Geometry: final body of the model. Coordinates: model frame, mm. A direction names the side the tool comes from. Round coordinates to 2 decimals unless told otherwise and drop trailing zeros. Order: outer loops, then holes, each group sorted by start corner. A loop starts at its lowest first (then second) coordinate and runs counter-clockwise, first axis right, second up. Notation, with made-up numbers: (-12, 30.25) - (33, 30.25) arc R21 ccw to (33, 52.25) - close; hole circle Ø5 at (9, -9.5). An arc over 180 degrees is marked (long way). Put each result on its own line as item: value. Start each with the question number.
(1) Pin query (flat end, axial travel): P1, Ø1.5, axis at x = 21, y = -4, coming from the -Z side; P2, Ø10.5, axis at x = 65.2, z = 33, coming from the -Y side; P3, Ø4, axis at x = 17, z = 40.5, coming from the -Y side; P4, Ø5, axis at x = 39.8, z = 33, coming from the -Y side (3 decimals). Return the tip coordinate at first contact, or that it passes through.
(2) Section C-C (z = 17.5). Output: boundary loops of the cut face in (x, y).
(3) Material intervals for L1, parallel to Y at x = 27.5, z = -1; L2, parallel to Z at x = 65, y = 5; L3, parallel to X at y = 5, z = 34, sorted ascending. Write a range as [from, to].
(4) Access query for faces 4 (the face through (1, 8.05, 1)), 5 (the face through (40, 14, 27.4)), 6 (the face through (1, 13, -13)). Directions: +Z, -Z, +X, -X, +Y, -Y. A direction counts if a zero-diameter tool reaches every point of the face in a straight line with its end or side. Return the directions, or none.
(5) Pull-direction query (X, two-part tool) for faces 1 (the face through (1, 1, 13)), 2 (the face through (70.072, 14.499, 30.239)), 3 (the face through (-90, 3, 24)); classes: released by +X, released by -X, zero draft, split by the parting line, or undercut.
(6) Section A-A (z = -5). Output: boundary loops of the cut face in (x, y).
from build123d import *

# Parameters (mm, degrees)
F1_DEPTH = 90
F2_W     = 6
F2_H     = 61
F3_DEPTH = 5
F4_R     = 3.25
F5_DEPTH = 30.001
F7_DEPTH = 7
F8_SIZE  = 0.99999
F9_SIZE  = 1


# Not quite as in the source:
# - a fillet or chamfer is up to 0.001 mm smaller than in the source, because OpenCascade refuses the exact size


with BuildPart() as f1:
    # F0 (on Right) → F1 (new body, symmetric)
    with BuildSketch(Plane.YZ):
        Polygon((-6.05, 13), (8.05, 13), (8.05, -13), (17.95, -13), (17.95, 48), (-12.05, 48), (-12.05, -13), (-8.05, -13), (-8.05, 14), (-6.05, 14), align=None)
    extrude(amount=F1_DEPTH, both=True)

    # F2 (on face) → F3 (join)
    with BuildSketch(Plane.XZ.offset(12.05)):
        with Locations((87, 17.5)):
            Rectangle(F2_W, F2_H)
    extrude(amount=F3_DEPTH)

    # F4 (on face) → F5 (cut, through all)
    with BuildSketch(Plane.XZ.offset(12.05)):
        with Locations((39.8, 33)):
            Circle(F4_R)
        with Locations((65.2, 33)):
            Circle(F4_R)
    extrude(amount=-F5_DEPTH, mode=Mode.SUBTRACT)

    # F6 (on face) → F7 (cut)
    with BuildSketch(Plane(origin=(0, 17.95, 0), x_dir=(-1, 0, 0), z_dir=(0, 1, 0))):
        Polygon((-61.9668384925, 38.6), (-68.4331615075, 38.6), (-71.6663230149, 33), (-68.4331615075, 27.4), (-61.9668384925, 27.4), (-58.7336769851, 33), align=None)
        Polygon((-36.5668384925, 38.6), (-43.0331615075, 38.6), (-46.2663230149, 33), (-43.0331615075, 27.4), (-36.5668384925, 27.4), (-33.3336769851, 33), align=None)
    extrude(amount=-F7_DEPTH, mode=Mode.SUBTRACT)

    # F8 (size 1 in the source; OpenCascade refuses exactly that, so slightly less here)
    f8_edges = [f1.edges().sort_by_distance(p)[0] for p in [
        (0, -6.05, 13),
    ]]
    chamfer(f8_edges, length=F8_SIZE)

    # F9
    f9_edges = [f1.edges().sort_by_distance(p)[0] for p in [
        (0, -8.05, -13),
        (0, 8.05, -13),
        (0, 17.95, -13),
        (-90, 13, -13),
        (-90, 8.05, 0),
        (90, 13, -13),
        (-3, -12.05, -13),
        (-90, -10.05, -13),
        (84, -14.55, -13),
        (90, -12.55, -13),
        (87, -17.05, -13),
        (-90, -12.05, 17.5),
        (-90, 17.95, 17.5),
        (-90, -8.05, 0.5),
        (90, 8.05, 0),
        (90, -8.05, 0.5),
        (90, 1.499995, 13),
        (-90, 1.499995, 13),
        (90, 0.45, 48),
        (90, 17.95, 17.5),
        (0, 17.95, 48),
        (-3, -12.05, 48),
        (-90, 2.95, 48),
        (87, -17.05, 48),
        (84, -14.55, 48),
        (90, -17.05, 17.5),
        (84, -17.05, 17.5),
    ]]
    chamfer(f9_edges, length=F9_SIZE)


solid = f1.part
Checks:
1. P1: stops at z = 13
1. P2: stops at y = -12.05
1. P3: stops at y = -12.05
1. P4: passes through
2. outline: (-90, -11.05) - (-89, -12.05) - (84, -12.05) - (84, -16.05) - (85, -17.05) - (89, -17.05) - (90, -16.05) - (90, 16.95) - (89, 17.95) - (-89, 17.95) - (-90, 16.95) - close
3. L1: y = [-12.05, -8.05], [8.05, 17.95]
3. L2: z = [13, 29.76], [36.24, 48]
3. L3: x = [-90, 36.71], [42.89, 62.11], [68.29, 90]
4. face 4: -Z, +X, -X
4. face 5: +Y
4. face 6: -Z, +X, -X, +Y, -Y
5. face 1: zero draft
5. face 2: undercut
5. face 3: released by -X
6. outline: (-90, -11.05) - (-89, -12.05) - (84, -12.05) - (84, -16.05) - (85, -17.05) - (89, -17.05) - (90, -16.05) - (90, -9.05) - (89, -8.05) - (-89, -8.05) - (-90, -9.05) - close; (-90, 9.05) - (-89, 8.05) - (89, 8.05) - (90, 9.05) - (90, 16.95) - (89, 17.95) - (-89, 17.95) - (-90, 16.95) - close
